Geometry check sheet. Reference: the model listing, model coordinates, mm. A direction names the side the tool comes from. Round coordinates to 2 decimals unless told otherwise and drop trailing zeros. Order: outer loops, then holes, each group sorted by start corner. A loop starts at its lowest first (then second) coordinate and runs counter-clockwise, first axis right, second up. Notation, with made-up numbers: M 65.25,-15.75 L 81.25,-15.75 A22 ccw 81.25,3.25 Z; hole C -33,-21.75 d4. An arc over 180 degrees is marked long. Return JSON: item names as keys, results as strings. Group by question number.
```python
from build123d import *

# Parameters (mm, degrees)
SKETCH_1_R          = 3
SKETCH_1_R_2        = 7
SKETCH_1_R_3        = 2.75
EXTRUDE_1_DEPTH     = 10
SKETCH_2_R          = 4.75
CUT_EXTRUDE_2_DEPTH = 6


with BuildPart() as part:
    # 草图1 → 拉伸1 (new body)
    with BuildSketch(Plane.XY):
        with BuildLine():
            Line((1190.508500062, 1011.627141179), (1190.508500062, 977.627141179))
            ThreePointArc((1190.508500062, 977.627141179), (1191.387179719, 975.505820835), (1193.508500062, 974.627141179))
            Line((1193.508500062, 974.627141179), (1227.508500062, 974.627141179))
            ThreePointArc((1227.508500062, 974.627141179), (1229.629820406, 975.505820835), (1230.508500062, 977.627141179))
            Line((1230.508500062, 977.627141179), (1230.508500062, 1011.627141179))
            ThreePointArc((1230.508500062, 1011.627141179), (1229.629820406, 1013.748461522), (1227.508500062, 1014.627141179))
            Line((1227.508500062, 1014.627141179), (1193.508500062, 1014.627141179))
            ThreePointArc((1193.508500062, 1014.627141179), (1191.387179719, 1013.748461522), (1190.508500062, 1011.627141179))
        make_face()
        with Locations((1218.758500062, 1002.877141179)):
            Circle(SKETCH_1_R, mode=Mode.SUBTRACT)
        with Locations((1218.758500062, 986.377141179)):
            Circle(SKETCH_1_R, mode=Mode.SUBTRACT)
        with Locations((1202.258500062, 1002.877141179)):
            Circle(SKETCH_1_R, mode=Mode.SUBTRACT)
        with Locations((1202.258500062, 986.377141179)):
            Circle(SKETCH_1_R, mode=Mode.SUBTRACT)
        with Locations((1210.508500062, 994.627141179)):
            Circle(SKETCH_1_R_2, mode=Mode.SUBTRACT)
        with Locations((1195.508500062, 1009.627141179)):
            Circle(SKETCH_1_R_3, mode=Mode.SUBTRACT)
        with Locations((1225.508500062, 1009.627141179)):
            Circle(SKETCH_1_R_3, mode=Mode.SUBTRACT)
        with Locations((1225.508500062, 979.627141179)):
            Circle(SKETCH_1_R_3, mode=Mode.SUBTRACT)
        with Locations((1195.508500062, 979.627141179)):
            Circle(SKETCH_1_R_3, mode=Mode.SUBTRACT)
    extrude(amount=EXTRUDE_1_DEPTH)

    # 草图2 → 拉伸2 (cut)
    with BuildSketch(Plane(origin=(0, 0, 0), x_dir=(-1, 0, 0), z_dir=(0, 0, -1))):
        with Locations((-1225.508500062, 1009.627141179)):
            Circle(SKETCH_2_R)
        with Locations((-1195.508500062, 1009.627141179)):
            Circle(SKETCH_2_R)
        with Locations((-1225.508500062, 979.627141179)):
            Circle(SKETCH_2_R)
        with Locations((-1195.508500062, 979.627141179)):
            Circle(SKETCH_2_R)
        with Locations((-1218.758500062, 1002.877141179)):
            Circle(SKETCH_2_R)
        with Locations((-1202.258500062, 1002.877141179)):
            Circle(SKETCH_2_R)
        with Locations((-1218.758500062, 986.377141179)):
            Circle(SKETCH_2_R)
        with Locations((-1202.258500062, 986.377141179)):
            Circle(SKETCH_2_R)
    extrude(amount=-CUT_EXTRUDE_2_DEPTH, mode=Mode.SUBTRACT)


solid = part.part
```
Q1. Section check D-D on x = 1203. Record the cut outline in (y, z).
Q2. Material ranges on line 1 along Y through (x, z) = (1202.5, 7.25); line 2 along Y through (x, z) = (1202, 0.5); line 3 along X through (y, z) = (994.5, 4), recorded low to high.
Q3. Section check B-B on y = 996. Record the cut outline in (x, z), plus the area to 3 significant figures.
Q4. Release check for a two-part mould opening along Y. For faces 1 (the face through (1229.606, 975.483, 4.93)), 2 (the face through (1194.912, 976.943, 7.972)), 3 (the face through (1201, 995, 0)) record: +Y half, -Y half, draft (parallel to the pull), parting line (faces both ways), or undercut.
Q5. Section check C-C on z = 0.5. Record the cut outline in (x, y).
Q6. Set-up check for faces 4 (the face through (1219, 983, 6)), 5 (the face through (1190.509, 995, 5)): record each of +Z, -Z, +X, -X, +Y, -Y from which the full face is reachable in a straight line by a thin tool's end or side.
Q7. Section check A-A on x = 1210.5. Record the cut outline in (y, z).
Q8. Depth check by flat-ended pin: pin 1 Ø3 at (x, y) = (1195.5, 977.5) entering from -Z; pin 2 Ø12.5 at (x, y) = (1210.51, 994.63) entering from +Z. Enter the tip coordinate at first touch or a pass-through.
Geometry check:
{
 "1": {"outline": "M 974.63,0 L 981.69,0 L 981.69,6 L 983.47,6 L 983.47,10 L 974.63,10 Z; M 989.28,6 L 991.07,6 L 991.07,0 L 998.19,0 L 998.19,6 L 999.97,6 L 999.97,10 L 989.28,10 Z; M 1005.78,6 L 1007.57,6 L 1007.57,0 L 1014.63,0 L 1014.63,10 L 1005.78,10 Z"},
 "2": {"line 1": "y = 974.63 to 983.39, 989.37 to 999.89, 1005.87 to 1014.63", "line 2": "y = 974.63 to 981.63, 991.12 to 998.13, 1007.62 to 1014.63", "line 3": "x = 1190.51 to 1203.51, 1217.51 to 1230.51"},
 "3": {"outline": "M 1190.51,0 L 1203.64,0 L 1203.64,10 L 1190.51,10 Z; M 1217.37,0 L 1230.51,0 L 1230.51,10 L 1217.37,10 Z", "area": "263 mm^2"},
 "4": {"face 1": "-Y half", "face 2": "undercut", "face 3": "draft"},
 "5": {"outline": "M 1190.51,977.63 A3 ccw 1193.51,974.63 L 1227.51,974.63 A3 ccw 1230.51,977.63 L 1230.51,1011.63 A3 ccw 1227.51,1014.63 L 1193.51,1014.63 A3 ccw 1190.51,1011.63 Z; hole C 1195.51,979.63 d9.5; hole C 1195.51,1009.63 d9.5; hole M 1205.1,990.18 A4.75 ccw long 1206.07,989.22 A7 ccw 1214.95,989.22 A4.75 ccw long 1215.92,990.18 A7 ccw 1215.92,999.07 A4.75 ccw long 1214.95,1000.04 A7 ccw 1206.07,1000.04 A4.75 ccw long 1205.1,999.07 A7 ccw Z; hole C 1225.51,979.63 d9.5; hole C 1225.51,1009.63 d9.5"},
 "6": {"face 4": "-Z", "face 5": "+Z, -Z, -X, +Y, -Y"},
 "7": {"outline": "M 974.63,0 L 987.63,0 L 987.63,10 L 974.63,10 Z; M 1001.63,0 L 1014.63,0 L 1014.63,10 L 1001.63,10 Z"},
 "8": {"pin 1": "stops at z = 6", "pin 2": "passes through"}
}
